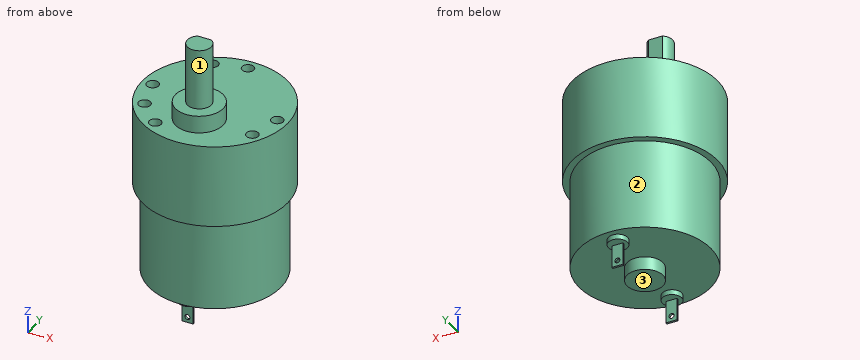
```python
from build123d import *

# Parameters (mm, degrees)
SKETCH1_R           = 18.161
BOSS_EXTRUDE1_DEPTH = 20.828
SKETCH2_R           = 16.51
BOSS_EXTRUDE2_DEPTH = 22.606
SKETCH3_R           = 4.5085
BOSS_EXTRUDE3_DEPTH = 3.302
SKETCH4_R           = 2.413
BOSS_EXTRUDE4_DEPTH = 1.27
SKETCH5_R           = 5.969
BOSS_EXTRUDE5_DEPTH = 4.3688
BOSS_EXTRUDE6_DEPTH = 15.24
SKETCH8_W           = 5.588
SKETCH8_H           = 2.794
SKETCH8_R           = 0.635
BOSS_EXTRUDE7_DEPTH = 0.254
CIRPATTERN1_COUNT   = 2
CIRPATTERN2_COUNT   = 12


with BuildPart() as part:
    # Sketch1 → Boss-Extrude1 (new body)
    with BuildSketch(Plane.XY):
        Circle(SKETCH1_R)
    extrude(amount=BOSS_EXTRUDE1_DEPTH)

    # Sketch2 → Boss-Extrude2 (add)
    with BuildSketch(Plane(origin=(0, 0, 0), x_dir=(-1, 0, 0), z_dir=(0, 0, -1))):
        Circle(SKETCH2_R)
    extrude(amount=BOSS_EXTRUDE2_DEPTH)

    # Sketch3 → Boss-Extrude3 (add)
    with BuildSketch(Plane(origin=(0, 0, -22.606), x_dir=(-1, 0, 0), z_dir=(0, 0, -1))):
        Circle(SKETCH3_R)
    extrude(amount=BOSS_EXTRUDE3_DEPTH)

    # Sketch4 → Boss-Extrude4 (add)
    with BuildSketch(Plane(origin=(0, 0, -22.606), x_dir=(-1, 0, 0), z_dir=(0, 0, -1))):
        with Locations((0, -12.7)):
            Circle(SKETCH4_R)
        with Locations((0, 12.7)):
            Circle(SKETCH4_R)
    extrude(amount=BOSS_EXTRUDE4_DEPTH)

    # Sketch5 → Boss-Extrude5 (add)
    with BuildSketch(Plane.XY.offset(20.828)):
        with Locations((0, -7.366)):
            Circle(SKETCH5_R)
    extrude(amount=BOSS_EXTRUDE5_DEPTH)

    # Sketch6 → Boss-Extrude6 (add)
    with BuildSketch(Plane.XY.offset(25.1968)):
        with BuildLine():
            Line((-1.715657017, -4.905), (1.715657017, -4.905))
            ThreePointArc((1.715657017, -4.905), (0, -10.366), (-1.715657017, -4.905))
        make_face()
    extrude(amount=BOSS_EXTRUDE6_DEPTH)

    # Sketch8 → Boss-Extrude7 (add, symmetric)
    with BuildSketch(Plane.ZX.offset(12.7)):
        with Locations((-26.67, 0)):
            Rectangle(SKETCH8_W, SKETCH8_H)
        with Locations((-28.067, 0)):
            Circle(SKETCH8_R, mode=Mode.SUBTRACT)
    boss_extrude7 = extrude(amount=BOSS_EXTRUDE7_DEPTH, both=True)

    # CirPattern1: Boss-Extrude7 ×2 about axis
    cirpattern1_axis = Axis((0, 0, 0), (0, 0, 1))
    for i in range(1, CIRPATTERN1_COUNT):
        add(boss_extrude7.rotate(cirpattern1_axis, i * 360 / CIRPATTERN1_COUNT))

    # Sketch12 → 3.0mm Dowel Hole1 (revolve, cut)
    with BuildSketch(Plane(origin=(0, 15.494, 20.828), x_dir=(0, -1, 0), z_dir=(1, 0, 0))):
        Polygon((0, 0), (0, 11.061290929), (1.5, 10.16), (1.5, 0), align=None)
    f_3_0mm_dowel_hole1 = revolve(axis=Axis((0, 15.494, 27.178), (0, 0, -1)), mode=Mode.SUBTRACT)

    # CirPattern2: 3.0mm Dowel Hole1 ×12 about axis, 5 skipped
    cirpattern2_axis = Axis((0, 0, 20.828), (0, 0, -1))
    add([f_3_0mm_dowel_hole1.rotate(cirpattern2_axis, i * 360 / CIRPATTERN2_COUNT) for i in range(1, CIRPATTERN2_COUNT) if i not in (1, 2, 5, 6, 10)], mode=Mode.SUBTRACT)


solid = part.part
```
Work out the finished part from the listing and answer in its coordinate system (mm). Face numbers are marked on the shaded views. A direction names the side the tool comes from. Give positions to 0.01 mm unless a question says otherwise; leave off trailing zeros. Write each loop counter-clockwise with the first axis right and the second up, starting at its lowest first coordinate (ties: lowest second). Pieces come first, ordered by that corner, then holes.
(1) Which of the six approach directions +Z, -Z, +X, -X, +Y, -Y give full straight-line access (tool end or side, diameter ignored) to the marked faces 1, 2 and 3?
Final values:
face 1: +Z
face 2: -Z
face 3: -Z, +X, -X
(2) The part is cut by section D-D on y = 3.5. Write down the section's boundary in (x, z).
Final values:
outline: (-17.82, 0) - (-16.13, 0) - (-16.13, -22.61) - (-2.84, -22.61) - (-2.84, -25.91) - (2.84, -25.91) - (2.84, -22.61) - (16.13, -22.61) - (16.13, 0) - (17.82, 0) - (17.82, 20.83) - (-17.82, 20.83) - close
(3) Straight lines are drawn through the part: line 1 (Z direction, x = 0, y = -12.6); line 2 (Z direction, x = 9, y = 13); line 3 (Z direction, x = -3.5, y = -7). For each, find the intervals that lie inside material, in ascending order.
Final values:
line 1: z = -29.46 to -28.7, -27.43 to 25.2
line 2: z = -22.61 to 20.83
line 3: z = -22.61 to 25.2
(4) Flat-ended cylindrical pins translate along their axes: pin 1 Ø4 at (x, y) = (-7.75, 13.42) entering from +Z; pin 2 Ø1.5 at (x, z) = (8, 16.5) entering from -Y; pin 3 Ø5 at (x, z) = (3, 6) entering from +Y; pin 4 Ø2 at (x, z) = (5, 32.5) entering from -Y. Find the tip coordinate at first contact, or state that the pin passes through.
Final values:
pin 1: stops at z = 20.83
pin 2: stops at y = -16.65
pin 3: stops at y = 18.15
pin 4: passes through
(5) The part is cut by section C-C on z = -19.5. Write down the section's boundary in (x, y), plus the area to 3 significant figures.
Final values:
outline: circle Ø33.02 at (0, 0)
area: 856 mm2
(6) The part is cut by section A-A on z = 12.5. Write down the section's boundary in (x, y), plus the area to 3 significant figures.
Final values:
outline: circle Ø36.32 at (0, 0); hole circle Ø3 at (-15.49, 0); hole circle Ø3 at (-13.42, -7.75); hole circle Ø3 at (-7.75, -13.42); hole circle Ø3 at (-7.75, 13.42); hole circle Ø3 at (0, 15.49); hole circle Ø3 at (13.42, -7.75); hole circle Ø3 at (15.49, 0)
area: 987 mm2
(7) The part is cut by section B-B on x = -10. Write down the section's boundary in (y, z), plus the area to 3 significant figures.
Final values:
outline: (-15.16, 0) - (-13.14, 0) - (-13.14, -22.61) - (13.14, -22.61) - (13.14, 0) - (15.16, 0) - (15.16, 20.83) - (-15.16, 20.83) - close
area: 1,230 mm2
